Answer from the drawing. Dimensions are ordinates in mm from the lowest x, y and z of the part. Round coordinates to 2 decimals unless told otherwise and drop trailing zeros. Write each loop counter-clockwise with the first axis right and the second up, starting at its lowest first coordinate (ties: lowest second). Pieces come first, ordered by that corner, then holes. Notation, with made-up numbers: (47, 79.5) - (89, 79.5) arc R11 cw to (89, 84.5) - close; hole circle Ø3 at (-27, -19). An arc over 180 degrees is marked (long way). One line per item, written item: value. Start each with the question number.
(1) The mould has two halves that part along X. Classify the marked faces 1, 2, 3 and 4: +X half, -X half, draft (parallel to the pull), parting line (faces both ways), or undercut.
(2) A cutting plane is placed at C-C, the plane z = 3.75. Determine the outline of the cut face in (x, y), plus the area to 3 significant figures.
(3) A cutting plane is placed at D-D, the plane z = 13.5. Determine the outline of the cut face in (x, y), plus the area to 3 significant figures.
(4) Flat-ended cylindrical pins translate along their axes: pin 1 Ø3 at (x, y) = (13.5, 7) entering from +Z; pin 2 Ø1.5 at (y, z) = (7, 13.5) entering from -X; pin 3 Ø6 at (y, z) = (5.5, 3.5) entering from -X; pin 4 Ø9 at (x, y) = (10, 10) entering from +Z. Find the tip coordinate at first contact, or state that the pin passes through.
(5) Find the intervals of material crossed by L1, parallel to Y at x = 10, z = 20; L2, parallel to Z at x = 9, y = 17.5; L3, parallel to X at y = 8, z = 2.5, in increasing order.
(6) A cutting plane is placed at A-A, the plane x = 10. Determine the outline of the cut face in (y, z), plus the area to 3 significant figures.
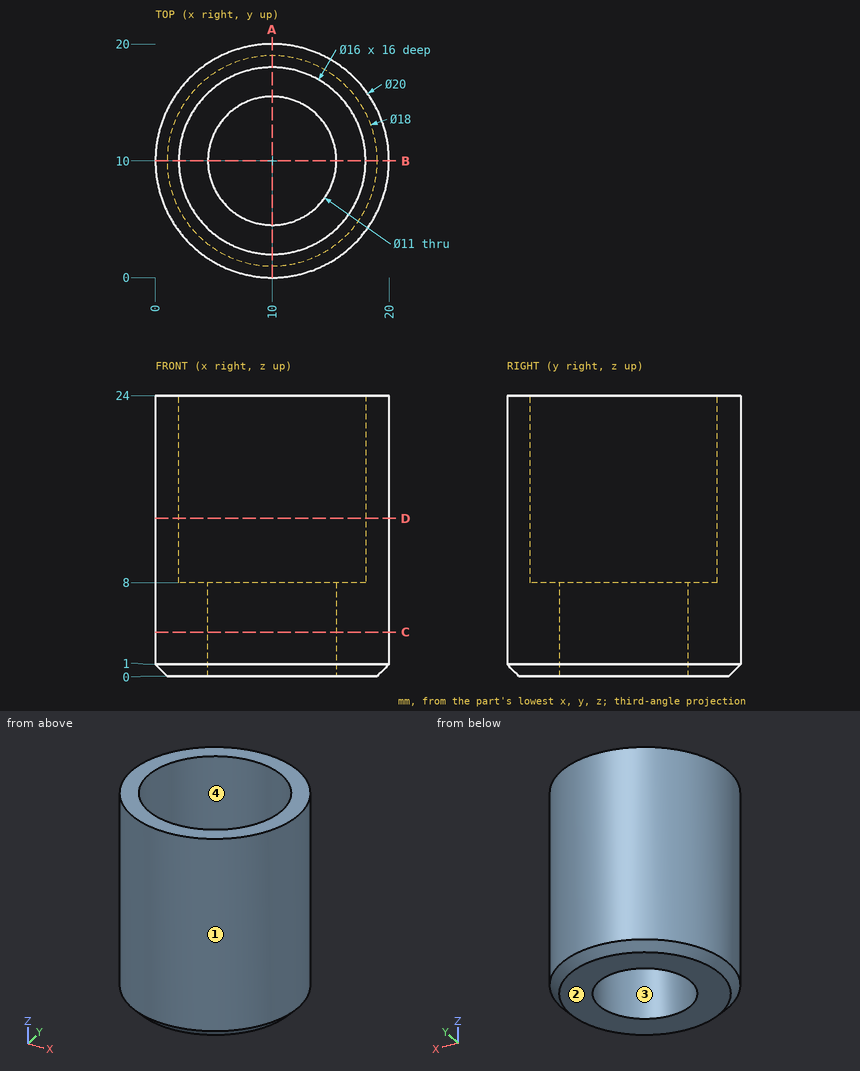
Here are the results:
1. face 1: parting line
1. face 2: draft
1. face 3: undercut
1. face 4: undercut
2. outline: circle Ø20 at (10, 10); hole circle Ø11 at (10, 10)
2. area: 219 mm²
3. outline: circle Ø20 at (10, 10); hole circle Ø16 at (10, 10)
3. area: 113 mm²
4. pin 1: z = 8
4. pin 2: x = 0.26
4. pin 3: x = 0.11
4. pin 4: through
5. L1: 0 to 2, 18 to 20
5. L2: 0 to 8
5. L3: 0.2 to 4.88, 15.12 to 19.8
6. outline: (0, 1) - (1, 0) - (4.5, 0) - (4.5, 8) - (2, 8) - (2, 24) - (0, 24) - close; (15.5, 0) - (19, 0) - (20, 1) - (20, 24) - (18, 24) - (18, 8) - (15.5, 8) - close
6. area: 135 mm²
